from build123d import *

# Parameters (mm, degrees)
SKETCH1_W           = 120
SKETCH1_H           = 90
BOSS_EXTRUDE1_DEPTH = 10
BOSS_EXTRUDE2_DEPTH = 10
SKETCH3_R           = 4
CUT_EXTRUDE1_DEPTH  = 10
CHAMFER2_SIZE       = 3
FILLET1_R           = 7
CUT_EXTRUDE2_DEPTH  = 7


with BuildPart() as part:
    # Sketch1 → Boss-Extrude1 (new body)
    with BuildSketch(Plane(origin=(0, 0, 0), x_dir=(1, 0, 0), z_dir=(0, 1, 0))):
        Rectangle(SKETCH1_W, SKETCH1_H)
    extrude(amount=BOSS_EXTRUDE1_DEPTH)

    # Sketch2 → Boss-Extrude2 (add)
    with BuildSketch(Plane(origin=(0, 10, 0), x_dir=(1, 0, 0), z_dir=(0, 1, 0))):
        with BuildLine():
            Line((60, -45), (-20, -45))
            Line((-20, -45), (-20, -29))
            ThreePointArc((-20, -29), (-49.247623411, 4.35052267), (-12.364838169, 28.994811876))
            Line((-12.364838169, 28.994811876), (60, 9.604711928))
            Line((60, 9.604711928), (60, -29))
            Line((60, -29), (60, -45))
        make_face()
    extrude(amount=BOSS_EXTRUDE2_DEPTH)

    # Cut-Sweep1: sweep along a path in Sketch4
    with BuildLine(Plane(origin=(0, 14, 0), x_dir=(1, 0, 0), z_dir=(0, 1, 0))) as cut_sweep1_path:
        Line((60, -32), (-20, -32))
        ThreePointArc((-20, -32), (-52.221957995, 4.742101247), (-11.588381034, 31.892589354))
        Line((-11.588381034, 31.892589354), (60, 12.710540469))
        Line((60, 12.710540469), (80.97534387, 7.090214018))
    # Sketch3 → Cut-Sweep1 (sweep, cut)
    with BuildSketch(Plane(origin=(60, 0, 0), x_dir=(0, 0, -1), z_dir=(1, 0, 0))):
        with Locations((-32, 14)):
            Circle(SKETCH3_R)
    sweep(path=cut_sweep1_path.line, mode=Mode.SUBTRACT)

    # Sketch5 → Cut-Extrude1 (cut)
    with BuildSketch(Plane(origin=(0, 20, 0), x_dir=(1, 0, 0), z_dir=(0, 1, 0))):
        with BuildLine():
            Line((-15, -18), (-15, -33))
            Line((-15, -33), (45, -33))
            Line((45, -33), (45, -23))
            Line((45, -23), (60, -23))
            Line((60, -23), (60, -1.783326057))
            Line((60, -1.783326057), (-15.211847666, 18.369627786))
            ThreePointArc((-15.211847666, 18.369627786), (-38.341729935, 2.914734556), (-20, -18))
            Line((-20, -18), (-15, -18))
        make_face()
    extrude(amount=-CUT_EXTRUDE1_DEPTH, mode=Mode.SUBTRACT)

    # Chamfer2
    chamfer2_edges = [part.edges().sort_by_distance(p)[0] for p in [
        (22.394076167, 10, -8.293150865),
        (-17.5, 10, 18),
        (-38.341729935, 10, -2.914734556),
    ]]
    chamfer(chamfer2_edges, length=CHAMFER2_SIZE)

    # Fillet1
    fillet1_edges = [part.edges().sort_by_distance(p)[0] for p in [
        (-17.5, 20, 18),
        (-38.341729935, 20, -2.914734556),
        (22.394076167, 20, -8.293150865),
        (52.5, 20, 23),
    ]]
    fillet(fillet1_edges, radius=FILLET1_R - 0.0001)  # a hair under: the kernel refuses the full size

    # Sketch6 → Cut-Extrude2 (cut)
    with BuildSketch(Plane(origin=(60, 0, 0), x_dir=(0, 0, -1), z_dir=(1, 0, 0))):
        Polygon((-32, 6.205771366), (-25.25, 10.102885683), (-25.25, 20), (-38.75, 20), (-38.75, 10.102885683), align=None)
    extrude(amount=-CUT_EXTRUDE2_DEPTH, mode=Mode.SUBTRACT)


solid = part.part
The listing builds one solid part. Answer for the finished solid, in the listing's coordinates (mm). A direction names the side the tool comes from. Coordinates: 2 decimals unless noted, no trailing zeros. Loops run counter-clockwise (first coordinate to the right, second up) from the corner with the lowest first, then second, coordinate; pieces in that order, holes last. Notation, with made-up numbers: (77, 41) -> (126, 41) arc R16 ccw to (126, 54) -> close; hole circle Ø4 at (-12.75, 16.25). An arc over 180 degrees is marked (long way). Answer in a Markdown table with one row per item. Add a question column.
1. Flat-ended cylindrical pins translate along their axes: P1, Ø11, axis at y = 16.5, z = 28.5, coming from the -X side; P2, Ø7, axis at y = 13, z = 35, coming from the +X side; P3, Ø14.5, axis at x = -2, z = 10.5, coming from the +Y side. Find the tip coordinate at first contact, or state that the pin passes through.
2. The part is cut by section A-A, the plane z = -31.5. Write down the section's boundary in (x, y), then the cut area to 3 significant figures.
3. Consider line 1 (Y direction, x = 21, z = 32); line 2 (Z direction, x = -37.5, y = 18.25); line 3 (Z direction, x = 38, y = 11). Determine where each line is inside the solid, lowest interval first. Write a range as [from, to].
4. Determine the mould class of faces 5 (the flat face through (53, 18, 34)), 6 (the flat face through (-1, 0, -1)), 7 (the flat face through (-20, 15, 39)), 8 (the flat face through (45, 15, 27)) for opening direction X: +X half, -X half, draft (parallel to the pull), parting line (faces both ways), or undercut.
5. For faces 1 (the cylindrical face through (22.384, 17.895, -10.362)), 2 (the flat face through (14, 10, 45)), 3 (the flat face through (57, 15, 38.75)), 4 (the flat face through (23.311, 18.299, -19.435)), determine the directions among +Z, -Z, +X, -X, +Y, -Y from which every point of the face is accessible in a straight line to the end or side of a thin tool.
Answer below:
| question | item | result |
|---|---|---|
| 1 | P1 | x = -37.83 |
| 1 | P2 | x = 53 |
| 1 | P3 | y = 10 |
| 2 | outline | (-60, 0) -> (60, 0) -> (60, 10) -> (-60, 10) -> close |
| 2 | area | 1,200 mm2 |
| 3 | line 1 | [0, 10] |
| 3 | line 2 | [-24.25, -11.87], [10.87, 23.25] |
| 3 | line 3 | [-15.5, -2.04], [34.65, 45] |
| 4 | face 5 | +X half |
| 4 | face 6 | draft |
| 4 | face 7 | -X half |
| 4 | face 8 | undercut |
| 5 | face 1 | +Y |
| 5 | face 2 | +Z, +X, -X, +Y, -Y |
| 5 | face 3 | +X, +Y |
| 5 | face 4 | -Z, +X, +Y |
